Input: part model. Units: mm. Frame: model coordinates. Give positions to 0.01 mm unless a question says otherwise; leave off trailing zeros. Write each loop counter-clockwise with the first axis right and the second up, starting at its lowest first coordinate (ties: lowest second). Pieces come first, ordered by that corner, then holes. Notation, with made-up numbers: (1.5, 73) - (12.5, 73) arc R35 ccw to (12.5, 105) - close; hole circle Ø3 at (16.25, 20.25). An arc over 180 degrees is marked (long way). Use a Markdown table: item, result. Add a question column.
1. Section query A-A, the plane y = 0. Return loops of the section in (x, z).
2. Material intervals for probe 1 along Y at (x, z) = (-7, 1.35); probe 2 along X at (y, z) = (4, 2.6); probe 3 along X at (y, z) = (-4, 0.65), sorted ascending.
3. Section query D-D, the plane z = 2.3. Count the separate pieces of the cut face and the enclosed holes in it, plus the area to 3 significant figures.
4. Section query C-C, the plane y = -5. Return loops of the section in (x, z), plus the area to 3 significant figures.
5. Pin query (flat end, axial travel): pin 1 (1.5 mm diameter, centred on y = 9, z = 1, fed in from +X); pin 2 (1.5 mm diameter, centred on x = 26, z = 2, fed in from +Y). Return the tip coordinate at first contact, or that it passes through.
6. Section query B-B, the plane x = -18.5. Return loops of the section in (y, z).
```python
from build123d import *

# Parameters (mm, degrees)
BOSS_EXTRUDE1_DEPTH = 3
CHAMFER1_SIZE       = 5
CUT_EXTRUDE1_DEPTH  = 5


with BuildPart() as part:
    # Sketch1 → Boss-Extrude1 (new body)
    with BuildSketch(Plane.XY):
        Polygon((22.5, -7.5), (22.5, -17.5), (-22.5, -17.5), (-22.5, -7.5), (-28.5, -7.5), (-28.5, 2.5), (-22.5, 2.5), (-22.5, 17.5), (22.5, 17.5), (22.5, 2.5), (28.5, 2.5), (28.5, -7.5), align=None)
    extrude(amount=BOSS_EXTRUDE1_DEPTH)

    # Chamfer1
    chamfer1_edges = [part.edges().sort_by_distance(p)[0] for p in [
        (-22.5, -17.5, 1.5),
        (-22.5, 17.5, 1.5),
        (22.5, 17.5, 1.5),
        (22.5, -17.5, 1.5),
    ]]
    chamfer(chamfer1_edges, length=CHAMFER1_SIZE)

    # Sketch2 → Cut-Extrude1 (cut)
    with BuildSketch(Plane.XY.offset(3)):
        with BuildLine():
            Line((-8, 1.5), (8, 1.5))
            ThreePointArc((8, 1.5), (9.5, 0), (8, -1.5))
            Line((8, -1.5), (-8, -1.5))
            ThreePointArc((-8, -1.5), (-9.5, 0), (-8, 1.5))
        make_face()
        with BuildLine():
            Line((-8, 6.5), (8, 6.5))
            ThreePointArc((8, 6.5), (9.5, 5), (8, 3.5))
            Line((8, 3.5), (-8, 3.5))
            ThreePointArc((-8, 3.5), (-9.5, 5), (-8, 6.5))
        make_face()
        with BuildLine():
            Line((-8, 11.5), (8, 11.5))
            ThreePointArc((8, 11.5), (9.5, 10), (8, 8.5))
            Line((8, 8.5), (-8, 8.5))
            ThreePointArc((-8, 8.5), (-9.5, 10), (-8, 11.5))
        make_face()
        with BuildLine():
            Line((-8, -3.5), (8, -3.5))
            ThreePointArc((8, -3.5), (9.5, -5), (8, -6.5))
            Line((8, -6.5), (-8, -6.5))
            ThreePointArc((-8, -6.5), (-9.5, -5), (-8, -3.5))
        make_face()
        with BuildLine():
            Line((-8, -8.5), (8, -8.5))
            ThreePointArc((8, -8.5), (9.5, -10), (8, -11.5))
            Line((8, -11.5), (-8, -11.5))
            ThreePointArc((-8, -11.5), (-9.5, -10), (-8, -8.5))
        make_face()
        with BuildLine():
            ThreePointArc((-12.715686471, 10.488674897), (-19.497563389, 0.236719508), (-13.143402946, -10.285689385))
            ThreePointArc((-13.143402946, -10.285689385), (-11.130912642, -9.614956372), (-11.801645656, -7.602466067))
            ThreePointArc((-11.801645656, -7.602466067), (-16.498199026, 0.174966593), (-11.485507392, 7.752498837))
            ThreePointArc((-11.485507392, 7.752498837), (-10.732508901, 9.735676407), (-12.715686471, 10.488674897))
        make_face()
        with BuildLine():
            ThreePointArc((12.715686471, 10.488674897), (19.497563389, 0.236719508), (13.143402946, -10.285689385))
            ThreePointArc((13.143402946, -10.285689385), (11.130912642, -9.614956372), (11.801645656, -7.602466067))
            ThreePointArc((11.801645656, -7.602466067), (16.498199026, 0.174966593), (11.485507392, 7.752498837))
            ThreePointArc((11.485507392, 7.752498837), (10.732508901, 9.735676407), (12.715686471, 10.488674897))
        make_face()
    extrude(amount=-CUT_EXTRUDE1_DEPTH, mode=Mode.SUBTRACT)


solid = part.part
```
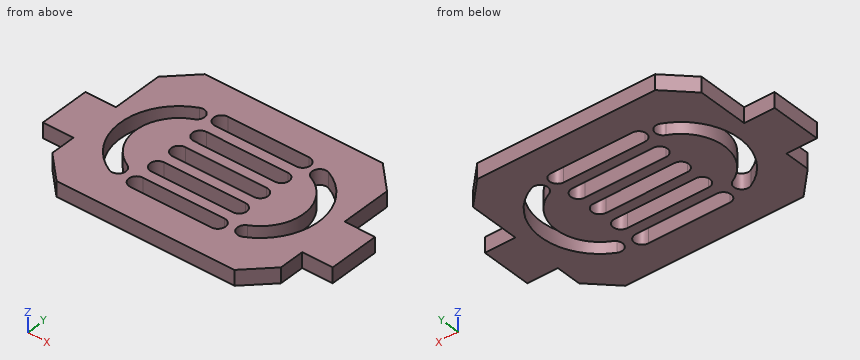
Result sheet:
| question | item | result |
|---|---|---|
| 1 | outline | (-28.5, 0) - (-19.5, 0) - (-19.5, 3) - (-28.5, 3) - close; (-16.5, 0) - (-9.5, 0) - (-9.5, 3) - (-16.5, 3) - close; (9.5, 0) - (16.5, 0) - (16.5, 3) - (9.5, 3) - close; (19.5, 0) - (28.5, 0) - (28.5, 3) - (19.5, 3) - close |
| 2 | probe 1 | y = -17.5 to -11.5, -8.5 to -6.5, -3.5 to -1.5, 1.5 to 3.5, 6.5 to 8.5, 11.5 to 17.5 |
| 2 | probe 2 | x = -22.5 to -18.78, -15.5 to -9.12, 9.12 to 15.5, 18.78 to 22.5 |
| 2 | probe 3 | x = -28.5 to -18.78, -15.5 to -9.12, 9.12 to 15.5, 18.78 to 28.5 |
| 3 | separate pieces | 1 |
| 3 | enclosed holes | 7 |
| 3 | area | 1,220 mm² |
| 4 | outline | (-28.5, 0) - (-18.36, 0) - (-18.36, 3) - (-28.5, 3) - close; (-14.87, 0) - (-9.5, 0) - (-9.5, 3) - (-14.87, 3) - close; (9.5, 0) - (14.87, 0) - (14.87, 3) - (9.5, 3) - close; (18.36, 0) - (28.5, 0) - (28.5, 3) - (18.36, 3) - close |
| 4 | area | 93.1 mm² |
| 5 | pin 1 | stops at x = 22.5 |
| 5 | pin 2 | stops at y = 2.5 |
| 6 | outline | (-16.5, 0) - (-4.69, 0) - (-4.69, 3) - (-16.5, 3) - close; (4.69, 0) - (16.5, 0) - (16.5, 3) - (4.69, 3) - close |
